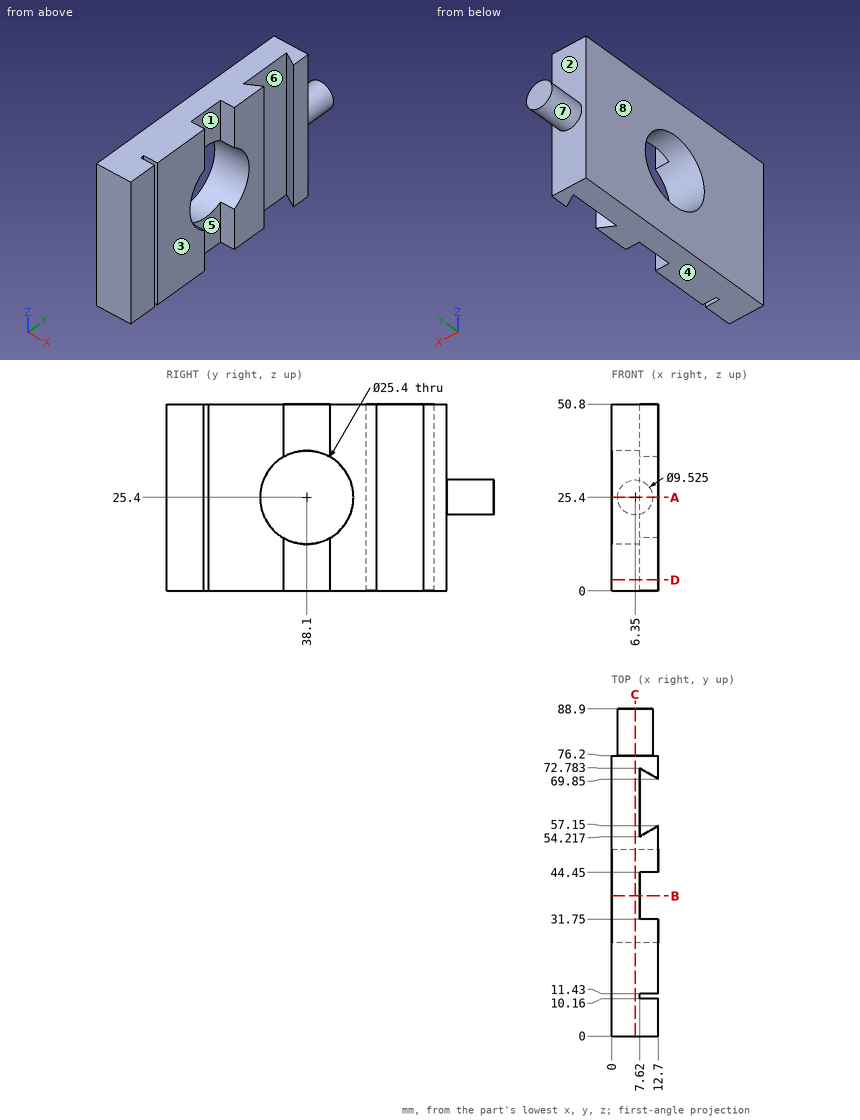
Answer from the drawing. Dimensions are ordinates in mm from the lowest x, y and z of the part. A direction names the side the tool comes from. Coordinates: 2 decimals unless noted, no trailing zeros. Order: outer loops, then holes, each group sorted by start corner. A loop starts at its lowest first (then second) coordinate and runs counter-clockwise, first axis right, second up. Notation, with made-up numbers: (57, 52) - (101, 52) arc R21 ccw to (101, 81) - close; hole circle Ø4 at (59, 2). An arc over 180 degrees is marked (long way). Answer as a JSON object with one key per item and string values. Group by question number.
Item 1: Section C-C (x = 6.35) is taken. Give the vertices of the cut face in (y, z), plus the area to 3 significant figures.
Item 2: Section B-B (y = 38.1) is taken. Give the vertices of the cut face in (x, z), plus the area to 3 significant figures.
Item 3: A tool of negligible diameter and unlimited length cuts with its end or side. For the marked faces 4, 5, 6, 7 and 8, from which of +Z, -Z, +X, -X, +Y, -Y can it reach the whole face along a straight path? Write none if from no direction.
Item 4: Section A-A (z = 25.4) is taken. Give the vertices of the cut face in (x, y).
Item 5: Consider probe 1 along Z at (x, y) = (2.5, 38.1); probe 2 along Y at (x, z) = (9.25, 6); probe 3 along Y at (x, z) = (10, 27). Determine where each line is inside the solid, lowest interval first. Write a range as from..to.
Item 6: Section D-D (z = 3) is taken. Give the vertices of the cut face in (x, y), plus the area to 3 significant figures.
Item 7: The mould has two halves that part along Y. Classify the marked faces 1, 2 and 3: +Y half, -Y half, draft (parallel to the pull), parting line (faces both ways), or undercut.
Item 8: Flat-ended cylindrical pins translate along their axes: P1, Ø5, axis at x = 8, z = 45.5, coming from the +Y side; P2, Ø0.6, axis at y = 10.5, z = 19.5, coming from the +X side. Find the tip coordinate at first contact, or state that the pin passes through.
Results are:
{
 "1": {"outline": "(0, 0) - (76.2, 0) - (76.2, 20.64) - (88.9, 20.64) - (88.9, 30.16) - (76.2, 30.16) - (76.2, 50.8) - (0, 50.8) - close; hole circle Ø25.4 at (38.1, 25.4)", "area": "3,490 mm^2"},
 "2": {"outline": "(0, 0) - (7.62, 0) - (7.62, 12.7) - (0, 12.7) - close; (0, 38.1) - (7.62, 38.1) - (7.62, 50.8) - (0, 50.8) - close", "area": "194 mm^2"},
 "3": {"face 4": "-Z, +X, -X, +Y, -Y", "face 5": "+Z, -Z, +X", "face 6": "+Z, -Z", "face 7": "+Y", "face 8": "+Z, -Z, -X, +Y, -Y"},
 "4": {"outline": "(0, 0) - (12.7, 0) - (12.7, 10.16) - (7.62, 10.16) - (7.62, 11.43) - (12.7, 11.43) - (12.7, 25.4) - (0, 25.4) - close; (0, 50.8) - (12.7, 50.8) - (12.7, 57.15) - (7.62, 54.22) - (7.62, 72.78) - (12.7, 69.85) - (12.7, 76.2) - (11.11, 76.2) - (11.11, 88.9) - (1.59, 88.9) - (1.59, 76.2) - (0, 76.2) - close"},
 "5": {"probe 1": "z = 0..12.7, 38.1..50.8", "probe 2": "y = 0..10.16, 11.43..31.75, 44.45..55.16, 71.84..76.2", "probe 3": "y = 0..10.16, 11.43..25.5, 50.7..55.59, 71.41..88.9"},
 "6": {"outline": "(0, 0) - (12.7, 0) - (12.7, 10.16) - (7.62, 10.16) - (7.62, 11.43) - (12.7, 11.43) - (12.7, 31.75) - (7.62, 31.75) - (7.62, 44.45) - (12.7, 44.45) - (12.7, 57.15) - (7.62, 54.22) - (7.62, 72.78) - (12.7, 69.85) - (12.7, 76.2) - (0, 76.2) - close", "area": "817 mm^2"},
 "7": {"face 1": "undercut", "face 2": "+Y half", "face 3": "draft"},
 "8": {"P1": "stops at y = 76.2", "P2": "stops at x = 7.62"}
}
